Here's how the part is built. I have some questions about the finished solid (model axes, mm). A direction names the side the tool comes from. Coordinates: 2 decimals unless noted, no trailing zeros. Write each loop counter-clockwise with the first axis right and the second up, starting at its lowest first coordinate (ties: lowest second). Pieces come first, ordered by that corner, then holes.
Item 1: If we mould it in two halves opening along Z, with no side actions, what happens to faces 6 (the face through (60.19, -3.54, 2.74)), 7 (the face through (3.875, -10.828, 4.486)), 8 (the face through (57.39, -7, 6)), 9 (the face through (57.19, -7.08, 7.33))? For each: pulls with the +Z half, pulls with the -Z half, needs draft (parallel to the pull), parting line crosses it, or undercut.
Item 2: I'm going to push flat-ended pins straight in: P1, Ø2.5, axis at x = 43.5, z = 4, coming from the +Y side; P2, Ø4, axis at x = 44.5, y = -6, coming from the +Z side; P3, Ø2, axis at y = -10, z = 1, coming from the -X side; P4, Ø1.5, axis at x = 40.5, z = 7, coming from the -Y side. Where does each tip first touch, or does it pass through?
Item 3: I want a section at A-A (y = -11.5). Please give me the cut outline in (x, z).
Item 4: I want a section at B-B (y = -1.5). Please give me the cut outline in (x, z).
Item 5: I want a section at C-C (x = 17). Please give me the cut outline in (y, z), and give its area (3 significant figures).
Item 6: Please list where these lines run through material, in increasing order: line 1 (X direction, y = -13, z = 2.5); line 2 (Z direction, x = 44, y = -13); line 3 (Y direction, x = 29.5, z = 1.75).
Item 7: For faces 1 (the face through (30, -7, 5.6)), 2 (the face through (30, -7, 0)), 3 (the face through (5, -7.185, 3)), 4 (the face through (55, -7.185, 2)), 5 (the face through (57, -14.37, 3)), which set-ups out of +Z, -Z, +X, -X, +Y, -Y let a thin tool reach every point of the face, with its end or its side?
from build123d import *

# Parameters (mm, degrees)
F1_DEPTH = 14.37
F0_R     = 2
F2_DEPTH = 7.185
F4_DEPTH = 14.57
F3_R     = 2
F5_DEPTH = 14.37
F7_DEPTH = 7.185


with BuildPart() as f1:
    # F0 (on Front) → F1 (new body)
    with BuildSketch(Plane.XZ):
        with BuildLine():
            Line((0, 5.6), (0, 0))
            Line((0, 0), (51.79, 0))
            ThreePointArc((51.79, 0), (53.7698989873, 0.8201010127), (54.59, 2.8))
            ThreePointArc((54.59, 2.8), (55.4101010127, 4.7798989873), (57.39, 5.6))
            Line((57.39, 5.6), (57.39, 6.7))
            ThreePointArc((57.39, 6.7), (57.1826506427, 7.3427867688), (56.6387730361, 7.7432436768))
            ThreePointArc((56.6387730361, 7.7432436768), (54.7187785908, 7.0266507051), (53.2475369646, 5.6))
            Line((53.2475369646, 5.6), (0, 5.6))
        make_face()
    extrude(amount=F1_DEPTH)



with BuildPart() as f1b:
    # F0 (on Front) → F1, piece 2 (new body)
    with BuildSketch(Plane.XZ):
        with Locations((57.39, 2.8)):
            Circle(F0_R)
    extrude(amount=F1_DEPTH)


with BuildPart() as f1_1:
    add(f1.part)

    add(f1b.part)  # F2 merges F1b
    # F0 (on Front) → F2 (join)
    with BuildSketch(Plane.XZ):
        with BuildLine():
            ThreePointArc((54.59, 2.8), (53.7698989873, 0.8201010127), (51.79, 0))
            Line((51.79, 0), (57.39, 0))
            ThreePointArc((57.39, 0), (60.19, 2.8), (57.39, 5.6))
            ThreePointArc((57.39, 5.6), (55.4101010127, 4.7798989873), (54.59, 2.8))
        make_face()
        with Locations((57.39, 2.8)):
            Circle(F0_R, mode=Mode.SUBTRACT)
    extrude(amount=F2_DEPTH)

    # F3 (on face) → F4 (join)
    with BuildSketch(Plane.XZ.offset(14.37)):
        with BuildLine():
            ThreePointArc((2.8, 7.8), (1.7, 6.6999999984), (2.8000000032, 5.6))
            ThreePointArc((2.8000000032, 5.6), (3.5778174604, 5.9221825418), (3.9, 6.7))
            ThreePointArc((3.9, 6.7), (3.5778174593, 7.4778174593), (2.8, 7.8))
        make_face()
        with BuildLine():
            ThreePointArc((3.9, 6.7), (3.5778174604, 5.9221825418), (2.8000000032, 5.6))
            Line((2.8000000032, 5.6), (6.9424630354, 5.6))
            ThreePointArc((6.9424630354, 5.6), (5.1452078799, 7.2158804332), (2.8, 7.8))
            ThreePointArc((2.8, 7.8), (3.5778174593, 7.4778174593), (3.9, 6.7))
        make_face()
    extrude(amount=-F4_DEPTH)

    # F3 (on face) → F5 (cut)
    with BuildSketch(Plane.XZ.offset(14.37)):
        with BuildLine():
            ThreePointArc((0, 2.8), (0.8201010138, 4.7798989885), (2.8000000032, 5.6))
            Line((2.8000000032, 5.6), (0, 5.6))
            Line((0, 5.6), (0, 2.8))
        make_face()
        with BuildLine():
            Line((0, 0), (2.8, 0))
            ThreePointArc((2.8, 0), (0.8201010127, 0.8201010127), (0, 2.8))
            Line((0, 2.8), (0, 0))
        make_face()
        with Locations((2.8, 2.8)):
            Circle(F3_R)
    extrude(amount=-F5_DEPTH, mode=Mode.SUBTRACT)

    # F6 (on face) → F7 (cut)
    with BuildSketch(Plane.XZ):
        with BuildLine():
            Line((5.6, 0), (5.6, 2.8))
            ThreePointArc((5.6, 2.8), (0.8201010127, 4.7798989873), (2.8, 0))
            Line((2.8, 0), (5.6, 0))
        make_face()
        with BuildLine():
            ThreePointArc((8.4, 0), (6.4201010127, 0.8201010127), (5.6, 2.8))
            Line((5.6, 2.8), (5.6, 0))
            Line((5.6, 0), (8.4, 0))
        make_face()
    extrude(amount=F7_DEPTH, mode=Mode.SUBTRACT)


solid = f1_1.part
Answer:
1. face 6: parting line crosses it
1. face 7: undercut
1. face 8: needs draft
1. face 9: pulls with the +Z half
2. P1: stops at y = 0
2. P2: stops at z = 5.6
2. P3: stops at x = 0.12
2. P4: passes through
3. outline: (2.8, 0) - (51.79, 0) arc R2.8 ccw to (54.59, 2.8) arc R2.8 cw to (57.39, 5.6) - (57.39, 6.7) arc R1.1 ccw to (56.64, 7.74) arc R5 ccw to (53.25, 5.6) - (6.94, 5.6) arc R5 ccw to (2.8, 7.8) arc R1.1 ccw to (2.8, 5.6) arc R2.8 ccw to start; circle Ø4 at (57.39, 2.8); hole circle Ø4 at (2.8, 2.8)
4. outline: (2.8, 5.6) arc R2.8 cw to (5.6, 2.8) arc R2.8 ccw to (8.4, 0) - (57.39, 0) arc R2.8 ccw to (57.39, 5.6) - (57.39, 6.7) arc R1.1 ccw to (56.64, 7.74) arc R5 ccw to (53.25, 5.6) - (6.94, 5.6) arc R5 ccw to (2.8, 7.8) arc R1.1 ccw to start
5. outline: (-14.37, 0) - (0, 0) - (0, 5.6) - (-14.37, 5.6) - close
5. area: 80.5 mm2
6. line 1: x = 0.02 to 0.82, 4.78 to 54.57, 55.41 to 59.37
6. line 2: z = 0 to 5.6
6. line 3: y = -14.37 to 0
7. face 1: +Z, +Y, -Y
7. face 2: -Z, +X, -X, +Y, -Y
7. face 3: -Z, -X, +Y
7. face 4: -Y
7. face 5: +Z, -Z, +X, -X, -Y
